Model file for the job. Use its own axes, mm. A direction names the side the tool comes from. Round coordinates to 2 decimals unless told otherwise and drop trailing zeros. Loops run counter-clockwise (first coordinate to the right, second up) from the corner with the lowest first, then second, coordinate; pieces in that order, holes last. Notation, with made-up numbers: (37.5, 72.25) - (55.5, 72.25) arc R17 ccw to (55.5, 76.25) - close; hole circle Ø3 at (28.5, -40). An arc over 180 degrees is marked (long way). Answer as a JSON object with one key per item and string values.
from build123d import *

# Parameters (mm, degrees)
SKETCH1_W           = 146
SKETCH1_H           = 140
BOSS_EXTRUDE1_DEPTH = 10
CUT_EXTRUDE1_DEPTH  = 10
SKETCH9_R           = 2
CUT_EXTRUDE4_DEPTH  = 20
SKETCH10_W          = 10
SKETCH10_H          = 10
CUT_EXTRUDE5_DEPTH  = 50
SKETCH12_R          = 3.175
BOSS_EXTRUDE2_DEPTH = 5
SKETCH14_W          = 14
SKETCH14_H          = 8
BOSS_EXTRUDE3_DEPTH = 5
SKETCH15_R          = 2
CUT_EXTRUDE6_DEPTH  = 20


with BuildPart() as part:
    # Sketch1 → Boss-Extrude1 (new body)
    with BuildSketch(Plane.XY):
        with Locations((73, 70)):
            Rectangle(SKETCH1_W, SKETCH1_H)
    extrude(amount=BOSS_EXTRUDE1_DEPTH)

    # Sketch4 → Cut-Extrude1 (cut)
    with BuildSketch(Plane.XY.offset(10)):
        with BuildLine():
            Line((14, 0), (132, 0))
            add(Edge.make_bspline(
                [(14, 0), (73, 260), (132, 0)],
                knots=[0, 0, 0, 1, 1, 1], degree=2))
        make_face()
    extrude(amount=-CUT_EXTRUDE1_DEPTH, mode=Mode.SUBTRACT)

    # Sketch9 → Cut-Extrude4 (cut)
    with BuildSketch(Plane.ZY):
        with Locations((5, 135)):
            Circle(SKETCH9_R)
        with Locations((5, 95)):
            Circle(SKETCH9_R)
    cut_extrude4 = extrude(amount=-CUT_EXTRUDE4_DEPTH, mode=Mode.SUBTRACT)

    # Sketch10 → Cut-Extrude5 (cut)
    with BuildSketch(Plane(origin=(0, 140, 0), x_dir=(1, 0, 0), z_dir=(0, 1, 0))):
        with Locations((5, -5)):
            Rectangle(SKETCH10_W, SKETCH10_H)
    cut_extrude5 = extrude(amount=-CUT_EXTRUDE5_DEPTH, mode=Mode.SUBTRACT)

    # Mirror3: Cut-Extrude4, Cut-Extrude5 across plane
    add(cut_extrude4.mirror(Plane.ZY.offset(-73)), mode=Mode.SUBTRACT)
    add(cut_extrude5.mirror(Plane.ZY.offset(-73)), mode=Mode.SUBTRACT)

    # Sketch12 → Boss-Extrude2 (add)
    with BuildSketch(Plane(origin=(0, 0, 0), x_dir=(1, 0, 0), z_dir=(0, 1, 0))):
        with BuildLine():
            Line((14, -10), (14, -14.625880325))
            ThreePointArc((14, -14.625880325), (14.374665781, -17.337511048), (15.470588235, -19.845950722))
            ThreePointArc((15.470588235, -19.845950722), (11.81635247, -30.105642379), (2.554902808, -24.375))
            ThreePointArc((2.554902808, -24.375), (2.224183895, -23.75), (1.562746067, -23.5))
            Line((1.562746067, -23.5), (1, -23.5))
            ThreePointArc((1, -23.5), (0.292893219, -23.207106781), (0, -22.5))
            Line((0, -22.5), (0, -10))
            Line((0, -10), (14, -10))
        make_face()
        with Locations(Location((9.5, -23.5, 0), (0, 0, 270))):
            Circle(SKETCH12_R, mode=Mode.SUBTRACT)
    boss_extrude2 = extrude(amount=BOSS_EXTRUDE2_DEPTH)

    # Mirror4: Boss-Extrude2 across plane
    add(boss_extrude2.mirror(Plane.ZY.offset(-73)))

    # Sketch14 → Boss-Extrude3 (add)
    with BuildSketch(Plane(origin=(0, 0, 0), x_dir=(1, 0, 0), z_dir=(0, 1, 0))):
        with Locations((7, 4)):
            Rectangle(SKETCH14_W, SKETCH14_H)
    boss_extrude3 = extrude(amount=BOSS_EXTRUDE3_DEPTH)

    # Mirror5: Boss-Extrude3 across plane
    add(boss_extrude3.mirror(Plane.ZY.offset(-73)))

    # Sketch15 → Cut-Extrude6 (cut)
    with BuildSketch(Plane.XY.offset(10)):
        with Locations((25, 135)):
            Circle(SKETCH15_R)
        with Locations((121, 135)):
            Circle(SKETCH15_R)
    extrude(amount=-CUT_EXTRUDE6_DEPTH, mode=Mode.SUBTRACT)


solid = part.part
1) Probe probe 1 along Z at (x, y) = (131, 95); probe 2 along Z at (x, y) = (10, 36); probe 3 along X at (y, z) = (61, 3.5). List the from-to ranges inside material, lowest first.
Values follow:
{"probe 1": "0 to 3, 7 to 10", "probe 2": "0 to 10", "probe 3": "0 to 30.02, 115.98 to 146"}
2) Drop flat-ended pins along their axis: P1, Ø6, axis at x = 114, z = -3.5, coming from the +Y side; P2, Ø8, axis at y = 114, z = 6, coming from the -X side; P3, Ø1.2, axis at y = 135, z = 4, coming from the -X side; P4, Ø7.5, axis at x = 9.5, z = 23.5, coming from the +Y side. Give the stop position or say it passes through.
Values follow:
{"P1": "through", "P2": "x = 10", "P3": "x = 20", "P4": "y = 5"}
3) Slice it at B-B on y = 135. List the corners of the cut face in (x, z), then the cut area to 3 significant figures.
Values follow:
{"outline": "(10, 0) - (23, 0) - (23, 10) - (10, 10) - (10, 7) - (20, 7) - (20, 3) - (10, 3) - close; (27, 0) - (119, 0) - (119, 10) - (27, 10) - close; (123, 0) - (136, 0) - (136, 3) - (126, 3) - (126, 7) - (136, 7) - (136, 10) - (123, 10) - close", "area": "1,100 mm²"}
4) Slice it at A-A on z = -2.5. List the corners of the cut face in (x, y), then the cut area to 3 significant figures.
Values follow:
{"outline": "(0, 0) - (14, 0) - (14, 5) - (0, 5) - close; (132, 0) - (146, 0) - (146, 5) - (132, 5) - close", "area": "140 mm²"}
5) Tool access for faces 1 (the flat face through (136, 115, 5)), 2 (the flat face through (20, 135, 5)), 3 (the flat face through (132, 2, -4)), 4 (the flat face through (5, 90, 5)), 5 (the cylindrical face through (14.364, 2.465, 17.3)): list every direction of +Z, -Z, +X, -X, +Y, -Y with a clear straight run to the whole face (end or side of a thin tool).
Values follow:
{"face 1": "+Z, -Z, +X, +Y", "face 2": "-X", "face 3": "-Z, +Y, -Y", "face 4": "+Z, -Z, -X, +Y", "face 5": "+Y, -Y"}
6) Two-plate mould, pull along Y, no slides. Class faces 6 (the cylindrical face through (11.98, 2.465, 30.046)), 7 (the flat face through (20, 95, 5)), 8 (the flat face through (8, 5, 18)): pulls with the +Y half, pulls with the -Y half, needs draft (parallel to the pull), parting line crosses it, or undercut.
Values follow:
{"face 6": "needs draft", "face 7": "undercut", "face 8": "pulls with the +Y half"}
